Could you check a few things on this model? Use its own coordinates, in mm. A direction names the side the tool comes from. Round coordinates to 2 decimals unless told otherwise and drop trailing zeros. Write each loop counter-clockwise with the first axis right and the second up, starting at its lowest first coordinate (ties: lowest second). Pieces come first, ordered by that corner, then holes. Notation, with made-up numbers: M 62.25,39 L 88.25,39 A18 ccw 88.25,44 Z; hole C -11.75,-37 d6. An arc over 180 degrees is marked long. One line per item, written item: value. Start each with the question number.
(1) If I drill on L1, parallel to X at y = 0, z = 3.7; L2, parallel to Z at x = -6.75, y = -2.25, over which ranges is the centre line in solid material (lowest first)?
(2) I want a section at D-D on y = -5.5. Please give me the cut outline in (x, z).
(3) Which directions (+Z, -Z, +X, -X, +Y, -Y) give clear straight access to the entire face, cutting with the end or side of a thin tool? Please do faces 5 (the face through (-1.73, 7.81, 0.76)), 6 (the face through (0, 0, 0)), 7 (the face through (-1.172, -8.923, 6.542)), 8 (the face through (0, 0, 9)), 9 (the face through (2, 2, 1.5)).
(4) I'm going to push flat-ended pins straight in: pin 1 Ø3 at (x, z) = (-2.5, 3.5) entering from +Y; pin 2 Ø1.5 at (x, z) = (3.5, 4.5) entering from +Y; pin 3 Ø1.5 at (y, z) = (1, 6) entering from +X. Where does each tip first touch, or does it pass through?
(5) Thinking about a two-plate mould opening in Z: for faces 1 (the face through (0, 7.3, 9.5)), 2 (the face through (0, 2, 3)), 3 (the face through (-1, -2, 4.5)), 4 (the face through (6.466, 2.681, 9.246)), which applies, released by +Z, released by -Z, zero draft, split by the parting line, or undercut?
(6) I want a section at A-A on y = 0. Please give me the cut outline in (x, z), and give its area (3 significant figures).
(7) I want a section at B-B on x = 5. Please give me the cut outline in (y, z) (3 decimals), and give its area (3 significant figures).
```python
from build123d import *


with BuildPart() as f1:
    # F0 (on Front) → F1 (revolve)
    with BuildSketch(Plane.XZ):
        Polygon((0, 1.5), (0, 0), (8, 0), (8, 1.5), (2, 1.5), align=None)
        Polygon((0, 9), (0, 1.5), (2, 1.5), (2, 4.5), (7, 4.5), (7, 3.5), (9, 3.5), (9, 9.5), (7, 9.5), (7, 9), align=None)
    revolve(axis=Axis((0, 0, 4.5), (0, 0, -1)))


solid = f1.part
```
Found:
1. L1: x = -9 to -7, -2 to 2, 7 to 9
1. L2: z = 0 to 1.5, 3.5 to 9.5
2. outline: M -7.12,3.5 L -4.33,3.5 L -4.33,4.5 L 4.33,4.5 L 4.33,3.5 L 7.12,3.5 L 7.12,9.5 L 4.33,9.5 L 4.33,9 L -4.33,9 L -4.33,9.5 L -7.12,9.5 Z; M -5.81,0 L 5.81,0 L 5.81,1.5 L -5.81,1.5 Z
3. face 5: -Z
3. face 6: -Z, +X, -X, +Y, -Y
3. face 7: +Z, -Z
3. face 8: +Z
3. face 9: none
4. pin 1: stops at y = 8.94
4. pin 2: stops at y = 8.57
4. pin 3: stops at x = 9
5. face 1: released by +Z
5. face 2: undercut
5. face 3: undercut
5. face 4: zero draft
6. outline: M -9,3.5 L -7,3.5 L -7,4.5 L -2,4.5 L -2,1.5 L -8,1.5 L -8,0 L 8,0 L 8,1.5 L 2,1.5 L 2,4.5 L 7,4.5 L 7,3.5 L 9,3.5 L 9,9.5 L 7,9.5 L 7,9 L -7,9 L -7,9.5 L -9,9.5 Z
6. area: 123 mm²
7. outline: M -7.483,3.5 L -4.899,3.5 L -4.899,4.5 L 4.899,4.5 L 4.899,3.5 L 7.483,3.5 L 7.483,9.5 L 4.899,9.5 L 4.899,9 L -4.899,9 L -4.899,9.5 L -7.483,9.5 Z; M -6.245,0 L 6.245,0 L 6.245,1.5 L -6.245,1.5 Z
7. area: 93.8 mm²
